Check sheet for the modelled part. Datum: model origin and axes. Units: mm. A direction names the side the tool comes from. Coordinates: 2 decimals unless noted, no trailing zeros. Order: outer loops, then holes, each group sorted by start corner. A loop starts at its lowest first (then second) coordinate and runs counter-clockwise, first axis right, second up.
Autodesk Inventor part; units mm, degrees
ref_plane "YZ Plane" through (0, 0, 0) normal (1, 0, 0) x (0, 1, 0)
ref_plane "XZ Plane" through (0, 0, 0) normal (0, 1, 0) x (-1, 0, 0)
ref_plane "XY Plane" through (0, 0, 0) normal (0, 0, 1) x (1, 0, 0)
sketch "Sketch1" plane through (0, 0, 0) normal (0, 1, 0) x (-1, 0, 0)
  circle A0 centre (0, 0) radius 4.9
  dimension "d0" = 9.8
extrude "Extrusion1" add sketch "Sketch1" along normal mid plane 20
sketch "Sketch2" plane through (0, 0, 0) normal (0, 1, 0) x (-1, 0, 0)
  circle A0 centre (0, 0) radius 7
  dimension "d3" = 14
extrude "Extrusion2" add sketch "Sketch2" along normal mid plane 4
sketch "Sketch3" plane through (0, 10, 0) normal (0, 1, 0) x (1, 0, 0)
  line L0 (-12, 0) -> (13, 0)
  line L1 (13, 0) -> (13, 11)
  line L2 (13, 11) -> (-12, 11)
  line L3 (-12, 11) -> (-12, 0)
  point P0 (0, 0)
extrude "Extrusion3" cut sketch "Sketch3" against normal blind 28
properties part number "wall_pin"
(1) Go/stop test with a flat-tipped pin: P1, Ø6, axis at x = -4, y = -3, coming from the +Z side. Record where the tip stops, or that it passes through.
Filled in:
P1: stops at z = 6.9
(2) Cross-section at B-B (z = 2.75). Enter the section's corners in (x, y).
Filled in:
outline: (-6.44, -2) - (-4.06, -2) - (-4.06, -10) - (4.06, -10) - (4.06, -2) - (6.44, -2) - (6.44, 2) - (4.06, 2) - (4.06, 10) - (-4.06, 10) - (-4.06, 2) - (-6.44, 2) - close
(3) Cross-section at A-A (x = -2.75). Enter the section's corners in (y, z).
Filled in:
outline: (-10, 0) - (10, 0) - (10, 4.06) - (2, 4.06) - (2, 6.44) - (-2, 6.44) - (-2, 4.06) - (-10, 4.06) - close
(4) Cross-section at C-C (y = 4). Enter the section's corners in (x, z).
Filled in:
outline: (-4.9, 0) - (4.9, 0) arc R4.9 ccw to start
(5) Cross-section at D-D (x = 0). Enter the section's corners in (y, z).
Filled in:
outline: (-10, 0) - (10, 0) - (10, 4.9) - (2, 4.9) - (2, 7) - (-2, 7) - (-2, 4.9) - (-10, 4.9) - close
(6) Tool access check on faces 1 (the flat face through (0, -10, 2)), 2 (the cylindrical face through (-0.1, -5.9, 4.9)), 3 (the flat face through (0.1, 2, 5.1)). Record the directions out of +Z, -Z, +X, -X, +Y, -Y that give a thin tool (end or side, any length) a straight path to the whole face; none if there is none.
Filled in:
face 1: +Z, -Z, +X, -X, -Y
face 2: +Z, -Y
face 3: +Z, +Y
(7) Thickness scan on probe 1 along Y at (x, z) = (4.5, 2.75); probe 2 along X at (y, z) = (1.75, 5); probe 3 along X at (y, z) = (8, 3). Record the ranges inside material, lowest first.
Filled in:
probe 1: y = -2 to 2
probe 2: x = -4.9 to 4.9
probe 3: x = -3.87 to 3.87
